Autodesk Inventor part; units mm, degrees
ref_plane "YZ Plane" through (0, 0, 0) normal (1, 0, 0) x (0, 1, 0)
ref_plane "XZ Plane" through (0, 0, 0) normal (0, 1, 0) x (-1, 0, 0)
ref_plane "XY Plane" through (0, 0, 0) normal (0, 0, 1) x (1, 0, 0)
sketch "Sketch1" plane through (0, 0, 0) normal (0, 1, 0) x (-1, 0, 0)
  line L0 (0, 30.3953) -> (0, -28.0277)
  circle A0 centre (0, 0) radius 100
  line L1 (95, 10.5) -> (40, 10.5)
  line L2 (40, 10.5) -> (40, 7.5)
  line L3 (40, 7.5) -> (95, 7.5)
  line L4 (95, 7.5) -> (95, 10.5)
  line L5 (95, -10.5) -> (40, -10.5)
  line L6 (40, -10.5) -> (40, -7.5)
  line L7 (40, -7.5) -> (95, -7.5)
  line L8 (95, -7.5) -> (95, -10.5)
  line L9 (0, 0) -> (75.0694, 0)
  line L10 (0, 0) -> (37.5347, 65.012)
  line L11 (0, 0) -> (-37.5347, 65.012)
  line L12 (0, 0) -> (-75.0694, 0)
  line L13 (0, 0) -> (-37.5347, -65.012)
  line L14 (0, 0) -> (37.5347, -65.012)
  circle A1 centre (0, 0) radius 35
  point P0 (20, 0)
  point P1 (10, 17.3205)
  point P2 (-10, 17.3205)
  point P3 (-20, 0)
  point P4 (-10, -17.3205)
  point P5 (10, -17.3205)
  dimension "d0" = 200
  dimension "t" = 3
  dimension "d2" = 55
  dimension "d3" = 40
  dimension "d4" = 15
  dimension "d21" = 360
  dimension "d27" = 70
extrude "Extrusion1" add sketch "Sketch1" along normal blind 6 contours A0 | L4 L3 L2 L1 | L5 L6 L7 L8 | L10 A1 L9 | L11 A1 L10 | L12 A1 L11 | L13 A1 L12 | L14 A1 L13 | L9 A1 L14
extrude "Extrusion3" cut sketch "Sketch1" along normal through all contours L4 L3 L2 L1 | L5 L6 L7 L8
pattern_circular "Circular Pattern1" count 6 over 360 about axis through (0, 0, 0) along (0, 1, 0) of "Extrusion3"
extrude "Extrusion5" cut sketch "Sketch1" along normal through all contours L10 A1 L9 | L11 A1 L10 | L12 A1 L11 | L13 A1 L12 | L14 A1 L13 | L9 A1 L14
sketch "Sketch2" plane through (0, 0, 0) normal (0, -1, 0) x (1, 0, 0)
  circle A0 centre (0, 0) radius 50
  dimension "d30" = 100
extrude "Extrusion6" add sketch "Sketch2" along normal blind 10
extrude "Extrusion7" cut sketch "Sketch1" against normal through all contours L10 A1 L9 | L11 A1 L10 | L12 A1 L11 | L13 A1 L12 | L14 A1 L13 | L9 A1 L14
equation "\"d5\" = 2 * t"
equation "\"d9\" = t"
equation "\"d28\" = t"
properties part number "rotor"
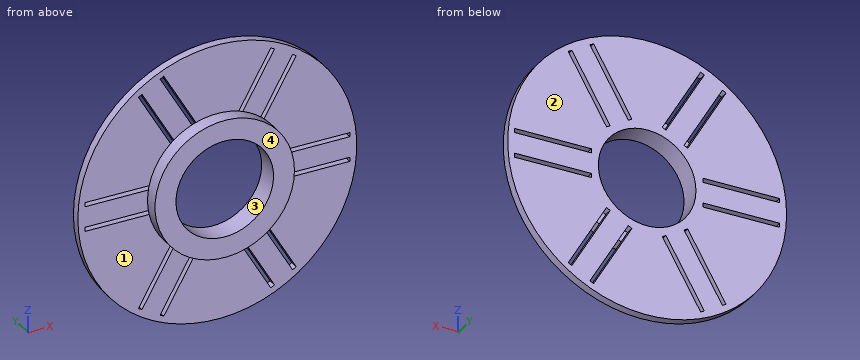
The model under review builds one solid part; all positions refer to its coordinate system, in mm. Face numbers are marked on the shaded views. A direction names the side the tool comes from. Round coordinates to 2 decimals unless told otherwise and drop trailing zeros. Loops run counter-clockwise (first coordinate to the right, second up) from the corner with the lowest first, then second, coordinate; pieces in that order, holes last. Notation, with made-up numbers: (-37.75, 24.25) -> (13.25, 24.25) arc R25 cw to (13.25, 42.25) -> close; hole circle Ø8 at (67.5, -20.5). An arc over 180 degrees is marked (long way). Answer as CSV lines item,"result".
1) Draft analysis for pull direction X (two halves, no side actions). For the marked faces 3 and 4, state which applies: pulls with the +X half, pulls with the -X half, needs draft (parallel to the pull), parting line crosses it, or undercut.
Geometry results:
face 3,"undercut"
face 4,"needs draft"
2) Add section A-A on x = 0. Write out the cut boundary in (y, z).
Geometry results:
outline,"(-10, -50) -> (0, -50) -> (0, -100) -> (6, -100) -> (6, -35) -> (-10, -35) -> close; (-10, 35) -> (6, 35) -> (6, 100) -> (0, 100) -> (0, 50) -> (-10, 50) -> close"
3) For P1, Ø1, axis at y = 1.5, z = 29.5, coming from the +X side; P2, Ø1.5, axis at x = -43.5, z = -9, coming from the +Y side; P3, Ø1.8, axis at x = 64, y = 3.5, coming from the +Z side, all flat-tipped, find the tip position at first contact; note any pin that passes through.
Geometry results:
P1,"stops at x = 95.7"
P2,"stops at y = 0"
P3,"stops at z = 77.58"
4) Tool access review of the marked faces 1 and 2: name each direction out of +Z, -Z, +X, -X, +Y, -Y from which nothing blocks a thin tool from reaching the whole face with its end or side.
Geometry results:
face 1,"-Y"
face 2,"+Z, -Z, +X, -X, +Y"
5) Add section C-C on y = -3. Write out the cut boundary in (x, z).
Geometry results:
outline,"circle Ø100 at (0, 0); hole circle Ø70 at (0, 0)"
6) Add section D-D on z = 74.5. Write out the cut boundary in (x, y).
Geometry results:
outline,"(-66.71, 0) -> (-55.14, 0) -> (-55.14, 6) -> (-66.71, 6) -> close; (-51.67, 0) -> (-34.35, 0) -> (-34.35, 6) -> (-51.67, 6) -> close; (-30.89, 0) -> (30.89, 0) -> (30.89, 6) -> (-30.89, 6) -> close; (34.35, 0) -> (51.67, 0) -> (51.67, 6) -> (34.35, 6) -> close; (55.14, 0) -> (66.71, 0) -> (66.71, 6) -> (55.14, 6) -> close"
7) Add section B-B on z = 0. Write out the cut boundary in (x, y).
Geometry results:
outline,"(-100, 0) -> (-50, 0) -> (-50, -10) -> (-35, -10) -> (-35, 6) -> (-100, 6) -> close; (35, -10) -> (50, -10) -> (50, 0) -> (100, 0) -> (100, 6) -> (35, 6) -> close"
8) To check wall thickness, follow line 1 along Z through (x, y) = (0, -6); line 2 along Z through (x, y) = (0, 1.25). State the ranges of each line that lie inside material, in increasing order. Write a range as from..to.
Geometry results:
line 1,"z = -50..-35, 35..50"
line 2,"z = -100..-35, 35..100"
